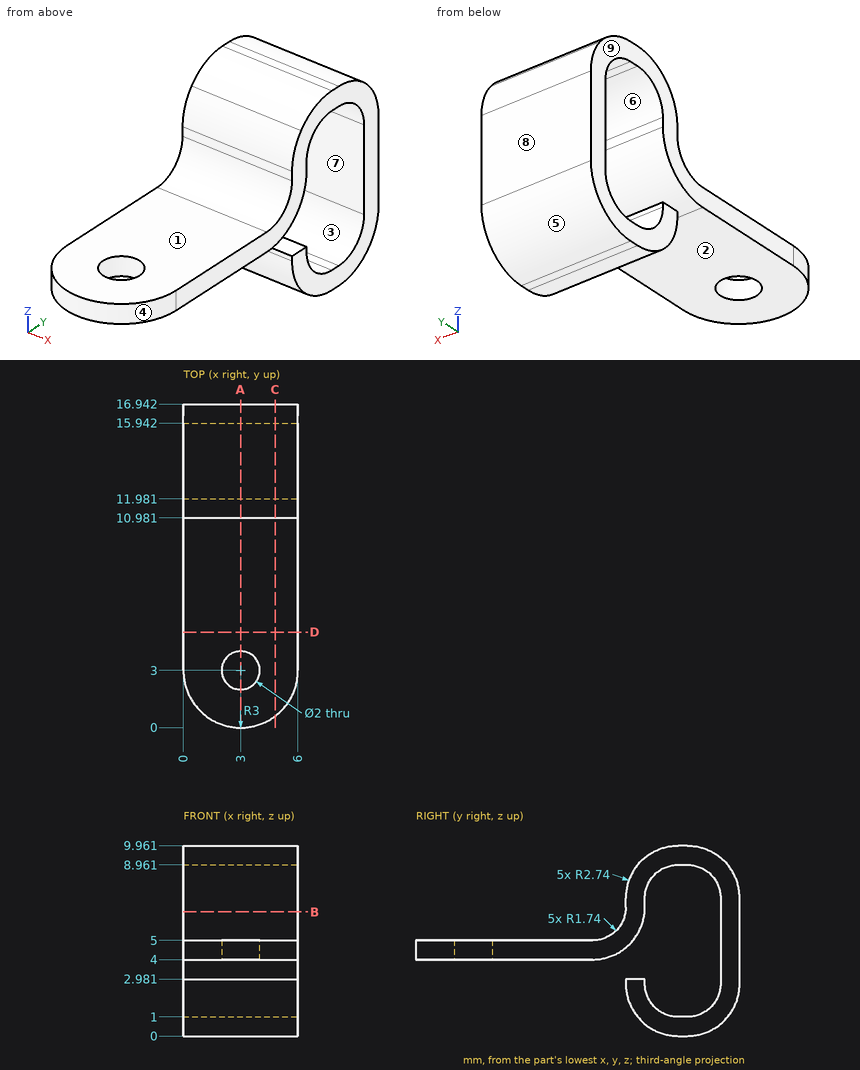
Job drawing, mm, ordinate dimensions from the low corner. One solid piece. A direction names the side the tool comes from. Give positions to 0.01 mm unless a question says otherwise; leave off trailing zeros. Order: outer loops, then holes, each group sorted by start corner. A loop starts at its lowest first (then second) coordinate and runs counter-clockwise, first axis right, second up. Notation, with made-up numbers: (6.5, 53) - (22.5, 53) arc R25 cw to (22.5, 80) - close; hole circle Ø11 at (-17.75, 30.5). An arc over 180 degrees is marked (long way). Answer in a Markdown table with one row per item.
1. Saw through at D-D, the plane y = 5. Give the cut face in (x, z).
Data:
| item | result |
|---|---|
| outline | (0, 4) - (6, 4) - (6, 5) - (0, 5) - close |
2. Saw through at C-C, the plane x = 4.8. Give the cut face in (y, z).
Data:
| item | result |
|---|---|
| outline | (0.6, 4) - (9.24, 4) arc R2.74 ccw to (11.98, 6.74) - (11.98, 7.22) arc R1.74 cw to (13.72, 8.96) - (14.2, 8.96) arc R1.74 cw to (15.94, 7.22) - (15.94, 2.74) arc R1.74 cw to (14.2, 1) - (13.72, 1) arc R1.74 cw to (11.98, 2.74) - (11.98, 2.98) - (10.98, 2.98) - (10.98, 2.74) arc R2.74 ccw to (13.72, 0) - (14.2, 0) arc R2.74 ccw to (16.94, 2.74) - (16.94, 7.22) arc R2.74 ccw to (14.2, 9.96) - (13.72, 9.96) arc R2.74 ccw to (10.98, 7.22) - (10.98, 6.74) arc R1.74 cw to (9.24, 5) - (0.6, 5) - close |
3. Probe probe 1 along Y at (x, z) = (3, 4.3) (1 decimal); probe 2 along Y at (x, z) = (2.8, 6.75); probe 3 along Y at (x, z) = (3, 4.4) (1 decimal). List the from-to ranges inside material, lowest first. Write a range as [from, to].
Data:
| item | result |
|---|---|
| probe 1 | y = [0, 2], [4, 10.5], [15.9, 16.9] |
| probe 2 | y = [10.98, 11.98], [15.94, 16.94] |
| probe 3 | y = [0, 2], [4, 10.7], [15.9, 16.9] |
4. Pull direction Y, two halves, no side cores. Call the marked faces 6, 7, 8 and 9: pulls with the +Y half, pulls with the -Y half, needs draft (parallel to the pull), parting line crosses it, or undercut.
Data:
| item | result |
|---|---|
| face 6 | undercut |
| face 7 | undercut |
| face 8 | pulls with the +Y half |
| face 9 | needs draft |
5. Tool access for the marked faces 1, 2, 3, 4 and 5: list every direction of +Z, -Z, +X, -X, +Y, -Y with a clear straight run to the whole face (end or side of a thin tool).
Data:
| item | result |
|---|---|
| face 1 | +Z, +X, -X, -Y |
| face 2 | -Z, +X, -X, -Y |
| face 3 | +X, -X |
| face 4 | +Z, -Z, -Y |
| face 5 | -Z, +X, -X, +Y |
6. Saw through at A-A, the plane x = 3. Give the cut face in (y, z).
Data:
| item | result |
|---|---|
| outline | (0, 4) - (2, 4) - (2, 5) - (0, 5) - close; (4, 4) - (9.24, 4) arc R2.74 ccw to (11.98, 6.74) - (11.98, 7.22) arc R1.74 cw to (13.72, 8.96) - (14.2, 8.96) arc R1.74 cw to (15.94, 7.22) - (15.94, 2.74) arc R1.74 cw to (14.2, 1) - (13.72, 1) arc R1.74 cw to (11.98, 2.74) - (11.98, 2.98) - (10.98, 2.98) - (10.98, 2.74) arc R2.74 ccw to (13.72, 0) - (14.2, 0) arc R2.74 ccw to (16.94, 2.74) - (16.94, 7.22) arc R2.74 ccw to (14.2, 9.96) - (13.72, 9.96) arc R2.74 ccw to (10.98, 7.22) - (10.98, 6.74) arc R1.74 cw to (9.24, 5) - (4, 5) - close |
7. Saw through at B-B, the plane z = 6.5. Give the cut face in (x, y).
Data:
| item | result |
|---|---|
| outline | (0, 10.96) - (6, 10.96) - (6, 11.97) - (0, 11.97) - close; (0, 15.94) - (6, 15.94) - (6, 16.94) - (0, 16.94) - close |
8. Flat gauge pins, fed straight in: pin 1 (3 mm diameter, centred on x = 2.5, y = 8, fed in from -Z); pin 2 (1.6 mm diameter, centred on x = 3, y = 3, fed in from +Z); pin 3 (2 mm diameter, centred on x = 3, z = 7.5, fed in from +Y); pin 4 (0.5 mm diameter, centred on x = 2, z = 7, fed in from -Y). Where does each tip first touch, or does it go through?
Data:
| item | result |
|---|---|
| pin 1 | stops at z = 4 |
| pin 2 | passes through |
| pin 3 | stops at y = 16.94 |
| pin 4 | stops at y = 10.98 |
